CAD build for the part. Positions are in the model's coordinates, mm. A direction names the side the tool comes from. Give positions to 0.01 mm unless a question says otherwise; leave off trailing zeros. Order: outer loops, then holes, each group sorted by start corner. A loop starts at its lowest first (then second) coordinate and runs counter-clockwise, first axis right, second up.
Item 1: Band-saw the part on B-B on x = 28. Give the cut face in (y, z).
Item 2: Which spindle directions (+Z, -Z, +X, -X, +Y, -Y) get a long thin tool onto all of the face, cutting with end or side? Do faces 1 (the cylindrical face through (23.8, -12.5, 23.4)), 2 (the flat face through (19, -15, 25)). Say none if no direction does.
Item 3: Flat gauge pins, fed straight in: P1, Ø1.5, axis at x = 24.5, z = 18.5, coming from the -Y side; P2, Ø3.5, axis at x = 4, z = 4, coming from the -Y side. Where does each tip first touch, or does it go through?
Item 4: Band-saw the part on D-D on x = 4. Give the cut face in (y, z).
Item 5: Band-saw the part on C-C on z = 4. Give the cut face in (x, y).
Item 6: Two-plate mould, pull along X, no slides. Class faces 3 (the flat face through (25, -1, 2)), 4 (the flat face through (49, -2, 25)), 5 (the flat face through (46, -8, 4)): released by +X, released by -X, zero draft, split by the parting line, or undercut.
Item 7: Wall check: L1, parallel to Z at x = 46, y = -9.5; L2, parallel to Z at x = 25, y = -11.55; L3, parallel to Z at x = 24.5, y = -5.75. Give the ranges that are in metal, low to high.
Item 8: Band-saw the part on A-A on z = 15. Give the cut face in (x, y).
```python
from build123d import *

# Parameters (mm, degrees)
F0_W      = 50
F0_H      = 50
F1_DEPTH  = 15
F2_W      = 10
F2_H      = 30
F3_DEPTH  = 1
F5_R      = 1.5
F6_DEPTH  = 4
F7_R      = 2.05
F8_DEPTH  = 7
F9_SIZE   = 3
F10_SIZE  = 3
F11_R     = 2.0899118634
F11_R_2   = 2.0672780913
F12_DEPTH = 12
F12_TAPER = 7


with BuildPart() as f1:
    # F0 (on Front) → F1 (new body)
    with BuildSketch(Plane.XZ):
        with Locations((25, 25)):
            Rectangle(F0_W, F0_H)
    extrude(amount=F1_DEPTH)

    # F2 (on face) → F3 (cut)
    with BuildSketch(Plane.XZ.offset(15)):
        with Locations((25, 25)):
            Rectangle(F2_W, F2_H)
    extrude(amount=-F3_DEPTH, mode=Mode.SUBTRACT)

    # F5 (on face) → F6 (cut)
    with BuildSketch(Plane.XZ.offset(15)):
        with Locations((25, 30)):
            Circle(F5_R)
        with Locations((25, 24.3)):
            Circle(F5_R)
        with Locations((25, 18.6)):
            Circle(F5_R)
    extrude(amount=-F6_DEPTH, mode=Mode.SUBTRACT)

    # F7 (on face) → F8 (cut)
    with BuildSketch(Plane.XZ.offset(15)):
        with Locations((46, 46)):
            Circle(F7_R)
        with Locations((46, 4)):
            Circle(F7_R)
        with Locations((4, 4)):
            Circle(F7_R)
        with Locations((4, 46)):
            Circle(F7_R)
    extrude(amount=-F8_DEPTH, mode=Mode.SUBTRACT)

    # F9
    f9_edges = [f1.edges().sort_by_distance(p)[0] for p in [
        (0, 0, 25),
        (25, 0, 0),
        (50, 0, 25),
        (25, 0, 50),
    ]]
    chamfer(f9_edges, length=F9_SIZE)

    # F10
    f10_edges = [f1.edges().sort_by_distance(p)[0] for p in [
        (0, -9, 50),
        (50, -9, 50),
        (50, -9, 0),
        (0, -9, 0),
    ]]
    chamfer(f10_edges, length=F10_SIZE)

    # F11 (on face) → F12 (cut)
    with BuildSketch(Plane(origin=(0, 0, 0), x_dir=(-1, 0, 0), z_dir=(0, 1, 0))):
        with Locations((-24.9610114843, 30.1139894873)):
            Circle(F11_R)
        with Locations((-24.8724594712, 18.6907239258)):
            Circle(F11_R_2)
    extrude(amount=-F12_DEPTH, taper=F12_TAPER, mode=Mode.SUBTRACT)


solid = f1.part
```
The answers:
1. outline: (-15, 0) - (-3, 0) - (0, 3) - (0, 47) - (-3, 50) - (-15, 50) - (-15, 40) - (-14, 40) - (-14, 10) - (-15, 10) - close
2. face 1: -Y
2. face 2: +Z, -Z, +X, -X, -Y
3. P1: stops at y = -11
3. P2: stops at y = -8
4. outline: (-15, 0) - (-3, 0) - (0, 3) - (0, 47) - (-3, 50) - (-15, 50) - (-15, 48.05) - (-8, 48.05) - (-8, 43.95) - (-15, 43.95) - (-15, 6.05) - (-8, 6.05) - (-8, 1.95) - (-15, 1.95) - close
5. outline: (0, -15) - (1.95, -15) - (1.95, -8) - (6.05, -8) - (6.05, -15) - (43.95, -15) - (43.95, -8) - (48.05, -8) - (48.05, -15) - (50, -15) - (50, -3) - (47, 0) - (3, 0) - (0, -3) - close
6. face 3: zero draft
6. face 4: released by +X
6. face 5: undercut
7. L1: z = 0 to 1.95, 6.05 to 43.95, 48.05 to 50
7. L2: z = 0 to 17.1, 20.1 to 22.8, 25.8 to 28.5, 31.5 to 50
7. L3: z = 0 to 17.38, 20 to 28.81, 31.42 to 50
8. outline: (0, -15) - (20, -15) - (20, -14) - (30, -14) - (30, -15) - (50, -15) - (50, -3) - (47, 0) - (3, 0) - (0, -3) - close
